Study the drawing (mm; zero at the part's minimum x, y, z) and answer. Give positions to 0.01 mm unless a question says otherwise; leave off trailing zeros. Write each loop counter-clockwise with the first axis right and the second up, starting at its lowest first coordinate (ties: lowest second). Pieces come first, ordered by that corner, then holes. Notation, with made-up numbers: (-2, 31.25) - (35, 31.25) arc R17 cw to (35, 60.25) - close; hole circle Ø8 at (-1.75, -27.75). An arc over 180 degrees is marked (long way). Answer as CSV lines item,"result".
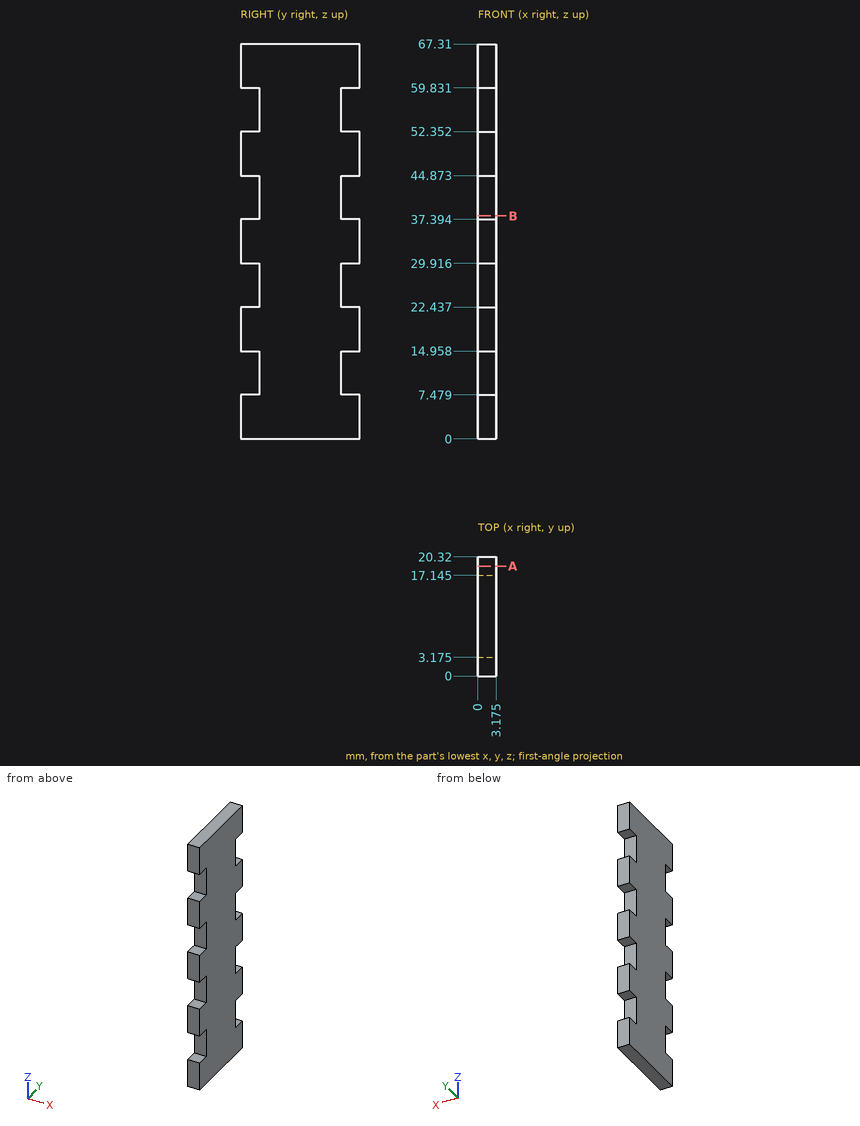
(1) A cutting plane is placed at B-B (z = 38). Write down the section's boundary in (x, y) (1 decimal).
Worked out:
outline,"(0, 3.2) - (3.2, 3.2) - (3.2, 17.1) - (0, 17.1) - close"
(2) Find the intervals of material crossed by L1, parallel to Z at x = 0.65, y = 17.75 (1 decimal); L2, parallel to Y at x = 2.65, z = 53 (1 decimal), in increasing order.
Worked out:
L1,"z = 0 to 7.5, 15 to 22.4, 29.9 to 37.4, 44.9 to 52.4, 59.8 to 67.3"
L2,"y = 3.2 to 17.1"
(3) A cutting plane is placed at A-A (y = 18.75). Write down the section's boundary in (x, z) (1 decimal).
Worked out:
outline,"(0, 0) - (3.2, 0) - (3.2, 7.5) - (0, 7.5) - close; (0, 15) - (3.2, 15) - (3.2, 22.4) - (0, 22.4) - close; (0, 29.9) - (3.2, 29.9) - (3.2, 37.4) - (0, 37.4) - close; (0, 44.9) - (3.2, 44.9) - (3.2, 52.4) - (0, 52.4) - close; (0, 59.8) - (3.2, 59.8) - (3.2, 67.3) - (0, 67.3) - close"
(4) Each of these flat-tipped pins is pushed along its axis until it touches: P1, Ø1.6, axis at x = 1.5, z = 26, coming from the +Y side (3 decimals); P2, Ø1.6, axis at x = 1, z = 10.5, coming from the -Y side (3 decimals). Where does it stop, or does it pass through?
Worked out:
P1,"stops at y = 17.145"
P2,"stops at y = 3.175"
